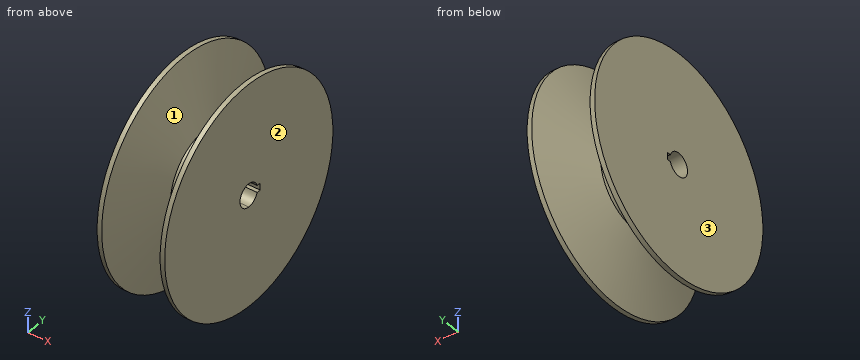
```python
from build123d import *

# Parameters (mm, degrees)
SKETCH1_W               = 3.175
SKETCH1_H               = 69.74205
CUT_EXTRUDE1_DEPTH      = 25.146
CUT_EXTRUDE1_DEPTH_BACK = 108.204


with BuildPart() as part:
    # Sketch1 → Revolve1 (revolve)
    with BuildSketch(Plane.XY, mode=Mode.PRIVATE) as revolve1_sk:
        Polygon((13.238453462, 31.037681507), (0, 76.09205), (0, 6.35), (22.013333333, 6.35), (40.64, 6.35), (40.64, 76.09205), (27.401546538, 31.037681507), align=None)
        with Locations((-1.5875, 41.221025)):
            Rectangle(SKETCH1_W, SKETCH1_H)
        with Locations((42.2275, 41.221025)):
            Rectangle(SKETCH1_W, SKETCH1_H)
    revolve(revolve1_sk.sketch.rotate(Axis((0, 0, 0), (1, 0, 0)), 90), axis=Axis((0, 0, 0), (1, 0, 0)))

    # Sketch2 → Cut-Extrude1 (cut, two sides: drawn at the far end of the back side and taken through both)
    with BuildSketch(Plane(origin=(43.815, 0, 0), x_dir=(0, 0, -1), z_dir=(1, 0, 0)).offset(-CUT_EXTRUDE1_DEPTH_BACK)):
        with BuildLine():
            Line((2.38125, 7.571892411), (2.38125, 5.886607549))
            ThreePointArc((2.38125, 5.886607549), (5.265141855, 3.549757914), (6.35, 0))
            ThreePointArc((6.35, 0), (-3.549757914, -5.265141855), (-2.38125, 5.886607549))
            Line((-2.38125, 5.886607549), (-2.38125, 7.571892411))
            ThreePointArc((-2.38125, 7.571892411), (-4.695888328, -6.399417088), (7.9375, 0))
            ThreePointArc((7.9375, 0), (6.399417088, 4.695888328), (2.38125, 7.571892411))
        make_face()
        with BuildLine():
            ThreePointArc((-2.38125, 5.886607549), (0, 6.35), (2.38125, 5.886607549))
            Line((2.38125, 5.886607549), (2.38125, 7.571892411))
            ThreePointArc((2.38125, 7.571892411), (0, 7.9375), (-2.38125, 7.571892411))
            Line((-2.38125, 7.571892411), (-2.38125, 5.886607549))
        make_face()
        with BuildLine():
            ThreePointArc((-2.38125, 7.571892411), (0, 7.9375), (2.38125, 7.571892411))
            Line((2.38125, 7.571892411), (2.38125, 10.31875))
            Line((2.38125, 10.31875), (-2.38125, 10.31875))
            Line((-2.38125, 10.31875), (-2.38125, 7.571892411))
        make_face()
        with BuildLine():
            Line((-2.38125, 5.55625), (2.38125, 5.55625))
            Line((2.38125, 5.55625), (2.38125, 5.886607549))
            ThreePointArc((2.38125, 5.886607549), (0, 6.35), (-2.38125, 5.886607549))
            Line((-2.38125, 5.886607549), (-2.38125, 5.55625))
        make_face()
    extrude(amount=CUT_EXTRUDE1_DEPTH + CUT_EXTRUDE1_DEPTH_BACK, mode=Mode.SUBTRACT)


solid = part.part
```
Input: part model. Units: mm. Frame: model coordinates. Face numbers are marked on the shaded views. Coordinates: 2 decimals unless noted, no trailing zeros. Loops run counter-clockwise (first coordinate to the right, second up) from the corner with the lowest first, then second, coordinate; pieces in that order, holes last. Notation, with made-up numbers: (25.5, 63) -> (51.5, 63) arc R21 cw to (51.5, 95) -> close; hole circle Ø9 at (-9.5, 81.5). An arc over 180 degrees is marked (long way). Use a Markdown table: item, result.
1) Cut plane C-C (x = 5). Return the cut outline in (y, z) (1 decimal), then the cut area to 3 significant figures.
Results found:
| item | result |
|---|---|
| outline | circle Ø118.2 at (0, 0); hole (7.6, -2.4) -> (10.3, -2.4) -> (10.3, 2.4) -> (7.6, 2.4) arc R7.9 ccw (long way) to start |
| area | 10,800 mm2 |
2) Material intervals for line 1 along Y through (x, z) = (15, 0); line 2 along X through (y, z) = (-46, -41.5) (3 decimals); line 3 along X through (y, z) = (-53.5, 22) (3 decimals), sorted ascending. Write a range as from..to.
Results found:
| item | result |
|---|---|
| line 1 | y = -31.04..-7.94, 10.32..31.04 |
| line 2 | x = -3.175..4.154, 36.486..43.815 |
| line 3 | x = -3.175..5.361, 35.279..43.815 |
3) Contact query for a flat-ended pin moving along its axis: pin 1 (2 mm diameter, centred on x = 23.5, y = 8.5, fed in from +Z). Output: stop coordinate, or through.
Results found:
| item | result |
|---|---|
| pin 1 | stops at z = 30.12 |
4) Cut plane A-A (z = 0). Return the cut outline in (x, y) (1 decimal), then the cut area to 3 significant figures.
Results found:
| item | result |
|---|---|
| outline | (-3.2, -76.1) -> (0, -76.1) -> (13.2, -31) -> (27.4, -31) -> (40.6, -76.1) -> (43.8, -76.1) -> (43.8, -7.9) -> (-3.2, -7.9) -> close; (-3.2, 10.3) -> (43.8, 10.3) -> (43.8, 76.1) -> (40.6, 76.1) -> (27.4, 31) -> (13.2, 31) -> (0, 76.1) -> (-3.2, 76.1) -> close |
| area | 3,820 mm2 |
5) Cut plane B-B (x = 30.5). Return the cut outline in (y, z) (1 decimal).
Results found:
| item | result |
|---|---|
| outline | circle Ø83.2 at (0, 0); hole (7.6, -2.4) -> (10.3, -2.4) -> (10.3, 2.4) -> (7.6, 2.4) arc R7.9 ccw (long way) to start |
6) Pull-direction query (X, two-part tool) for the marked faces 1, 2 and 3; classes: released by +X, released by -X, zero draft, split by the parting line, or undercut.
Results found:
| item | result |
|---|---|
| face 1 | undercut |
| face 2 | released by +X |
| face 3 | released by -X |
